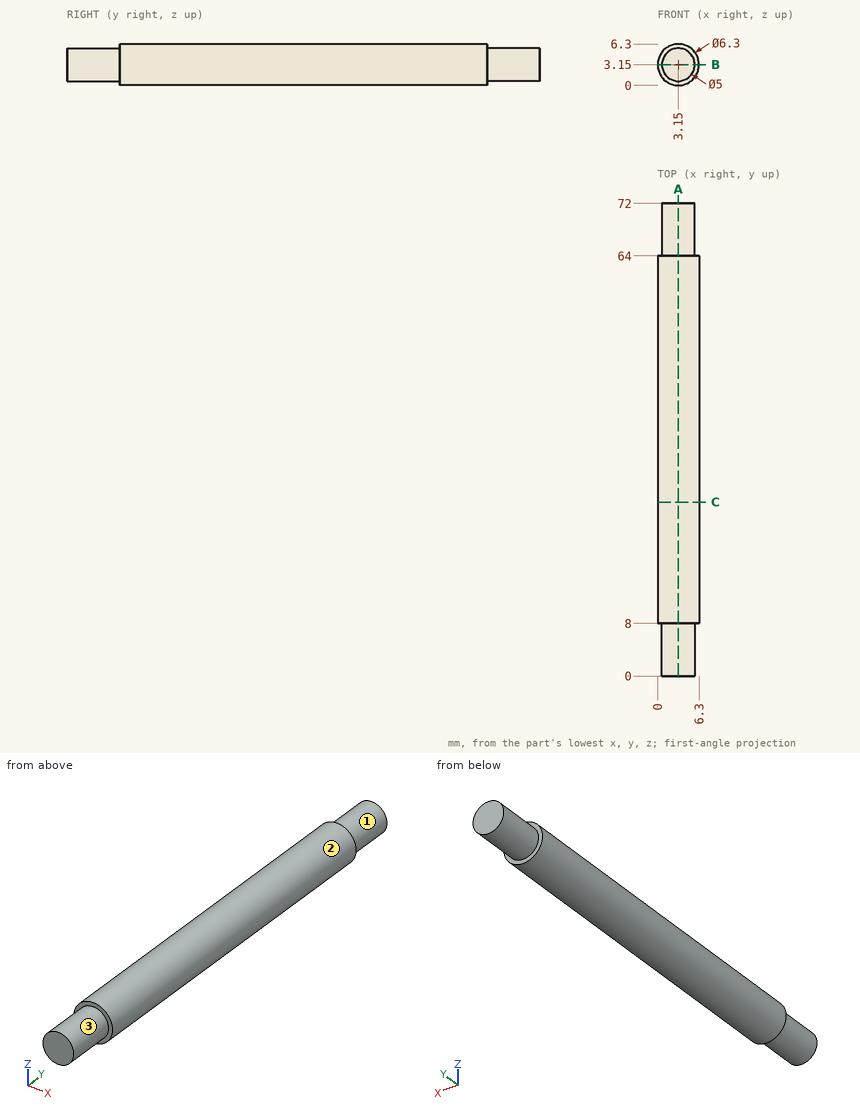
Geometry check sheet. Reference: drawing and pictorial views, mm from the part's lowest x, y, z. A direction names the side the tool comes from. Give positions to 0.01 mm unless a question says otherwise; leave off trailing zeros. Order: outer loops, then holes, each group sorted by start corner. A loop starts at its lowest first (then second) coordinate and runs counter-clockwise, first axis right, second up. Notation, with made-up numbers: (79.5, -22.5) -> (122.5, -22.5) arc R9 cw to (122.5, -10.5) -> close; hole circle Ø6 at (29, 65). An arc over 180 degrees is marked (long way). Write each question's results on one line, items separated by ' | '. Start each with the question number.
(1) Sectioned sample at B-B (z = 3.15). Enter the section's corners in (x, y), plus the area to 3 significant figures.
(2) Gauge pin test, flat ends, axial feed: P1, Ø1, axis at x = 2, z = 3.5, coming from the -Y side; P2, Ø1.5, axis at x = 5, y = 18, coming from the +Z side; P3, Ø2, axis at y = 54, z = 5, coming from the -X side. Record the tip position at first contact, or that the pin passes through.
(3) Sectioned sample at C-C (y = 26.5). Enter the section's corners in (x, z).
(4) Sectioned sample at A-A (x = 3.15). Enter the section's corners in (y, z), plus the area to 3 significant figures.
(5) Scan lines: line 1 (Z direction, x = 3, y = 18); line 2 (Y direction, x = 0.5, z = 3.75). Record each from-to range of solid material in increasing order.
(6) Access from +Z, -Z, +X, -X, +Y, -Y to the whole of each face (thin tool, end or side, straight path). Record for the marked faces 1, 2 and 3.
Answer below:
1) outline: (0, 8) -> (0.65, 8) -> (0.65, 0) -> (5.65, 0) -> (5.65, 8) -> (6.3, 8) -> (6.3, 64) -> (5.65, 64) -> (5.65, 72) -> (0.65, 72) -> (0.65, 64) -> (0, 64) -> close | area: 433 mm2
2) P1: y = 0 | P2: z = 6.1 | P3: x = 0.12
3) outline: circle Ø6.3 at (3.15, 3.15)
4) outline: (0, 0.65) -> (8, 0.65) -> (8, 0) -> (64, 0) -> (64, 0.65) -> (72, 0.65) -> (72, 5.65) -> (64, 5.65) -> (64, 6.3) -> (8, 6.3) -> (8, 5.65) -> (0, 5.65) -> close | area: 433 mm2
5) line 1: 0 to 6.3 | line 2: 8 to 64
6) face 1: +Y | face 2: +Y, -Y | face 3: -Y
